Check sheet for the modelled part. Datum: model origin and axes. Units: mm. Face numbers are marked on the shaded views. A direction names the side the tool comes from. Round coordinates to 2 decimals unless told otherwise and drop trailing zeros. Loops run counter-clockwise (first coordinate to the right, second up) from the corner with the lowest first, then second, coordinate; pieces in that order, holes last. Notation, with made-up numbers: (2, -8) - (17, -8) arc R20 ccw to (17, 31) - close; hole circle Ø9 at (20.5, 36.5). An arc over 180 degrees is marked (long way). Return JSON: item names as keys, results as strings.
from build123d import *

# Parameters (mm, degrees)
REVOLVE1_ANGLE           = 180
BOSS_EXTRUDE1_REACH      = 58.967
BOSS_EXTRUDE1_END_RADIUS = 40
SKETCH3_R                = 5.5
CUT_EXTRUDE1_DEPTH       = 61.16851336
SKETCH4_R                = 3
CUT_EXTRUDE2_DEPTH       = 61.16851336
CUT_EXTRUDE3_DEPTH       = 61.093676973
CUT_EXTRUDE3_DEPTH_BACK  = 61.093676973
SKETCH5_W                = 18.19644254
SKETCH5_H                = 2.5
SKETCH5_W_2              = 19.029010645
CHAMFER1_SIZE            = 2
FILLET1_R                = 1


with BuildPart() as part:
    # Sketch1 → Revolve1 (revolve)
    with BuildSketch(Plane(origin=(0, 0, 0), x_dir=(1, 0, 0), z_dir=(0, 1, 0))):
        with BuildLine():
            Line((-20, 20.5), (-20, -20.5))
            Line((-20, -20.5), (-25, -20.5))
            Line((-25, -20.5), (-25, -17.5))
            Line((-25, -17.5), (-35.968736425, -17.5))
            ThreePointArc((-35.968736425, -17.5), (-40, 0), (-35.968736425, 17.5))
            Line((-35.968736425, 17.5), (-25, 17.5))
            Line((-25, 17.5), (-25, 20.5))
            Line((-25, 20.5), (-20, 20.5))
        make_face()
    revolve(axis=Axis((0, 0, 0), (0, 0, -1)), revolution_arc=REVOLVE1_ANGLE)

    # Boss-Extrude1: up to this sphere (the profile starts outside it)
    boss_extrude1_end = Location((0, 0, 0)) * Sphere(BOSS_EXTRUDE1_END_RADIUS, mode=Mode.PRIVATE)
    # Sketch2 → Boss-Extrude1 (add, up to the surface)
    with BuildSketch(Plane(origin=(0, 35, 0), x_dir=(-1, 0, 0), z_dir=(0, -1, 0)), mode=Mode.PRIVATE) as boss_extrude1_sk1:
        with BuildLine():
            Line((30, 9), (17.860571099, 9))
            ThreePointArc((17.860571099, 9), (20, 0), (17.860571099, -9))
            Line((17.860571099, -9), (30, -9))
            ThreePointArc((30, -9), (39, 0), (30, 9))
        make_face()
    boss_extrude1_tool1 = extrude(boss_extrude1_sk1.sketch, amount=BOSS_EXTRUDE1_REACH, mode=Mode.PRIVATE) - boss_extrude1_end
    boss_extrude1 = boss_extrude1_tool1.solids().sort_by_distance((-28.288022, 35, 0))[0]
    add(boss_extrude1)

    # Sketch3 → Cut-Extrude1 (cut, through all)
    with BuildSketch(Plane.XZ):
        with Locations(Location((-30, 0, 0), (0, 0, 270))):
            Circle(SKETCH3_R)
    cut_extrude1 = extrude(amount=-CUT_EXTRUDE1_DEPTH, mode=Mode.SUBTRACT)

    # Mirror1: Boss-Extrude1, Cut-Extrude1 across plane
    add(boss_extrude1.mirror(Plane(origin=(0, 0, 0), x_dir=(0, 0, 1), z_dir=(1, 0, 0))))
    add(cut_extrude1.mirror(Plane(origin=(0, 0, 0), x_dir=(0, 0, 1), z_dir=(1, 0, 0))), mode=Mode.SUBTRACT)

    # Sketch4 → Cut-Extrude2 (cut, through all)
    with BuildSketch(Plane.XZ):
        with Locations(Location((0, 0, 0), (0, 0, 270))):
            Circle(SKETCH4_R)
    extrude(amount=-CUT_EXTRUDE2_DEPTH, mode=Mode.SUBTRACT)

    # Sketch5 → Cut-Extrude3 (cut, two sides: drawn at the far end of the back side and taken through both)
    with BuildSketch(Plane.XY.offset(-CUT_EXTRUDE3_DEPTH_BACK)):
        with Locations((-39.09822127, 1.25)):
            Rectangle(SKETCH5_W, SKETCH5_H)
        with Locations((39.514505322, 1.25)):
            Rectangle(SKETCH5_W_2, SKETCH5_H)
    extrude(amount=CUT_EXTRUDE3_DEPTH + CUT_EXTRUDE3_DEPTH_BACK, mode=Mode.SUBTRACT)

    # Chamfer1
    chamfer1_edges = [part.edges().sort_by_distance(p)[0] for p in [
        (0, 20, -20.5),
        (0, 20, 20.5),
    ]]
    chamfer(chamfer1_edges, length=CHAMFER1_SIZE)

    # Fillet1
    fillet1_edges = [part.edges().sort_by_distance(p)[0] for p in [
        (0, 25, 20.5),
        (0, 25, 17.5),
        (0, 25, -17.5),
        (0, 25, -20.5),
    ]]
    fillet(fillet1_edges, radius=FILLET1_R)


solid = part.part
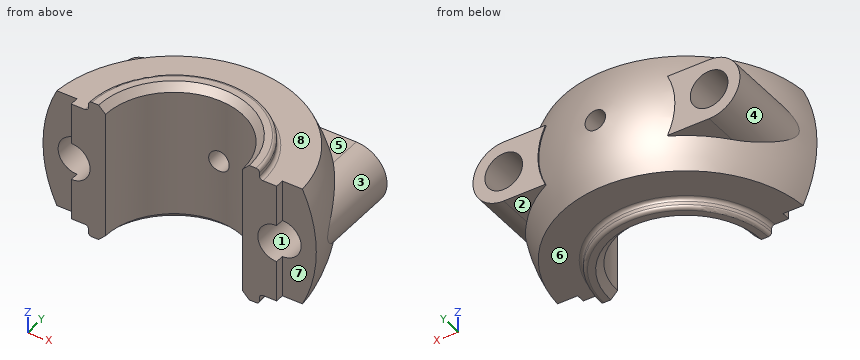
Q1. Sectioned sample at C-C (y = 14.5). State how many separate pieces and enclosed holes the cut face has, plus the area to 3 significant figures.
Answer key:
{"separate pieces": "2", "enclosed holes": "2", "area": "1,450 mm²"}
Q2. Sectioned sample at A-A (x = 0). Enter the section's corners in (y, z).
Answer key:
{"outline": "(20, -18.5) - (22, -20.5) - (24, -20.5) arc R1 ccw to (25, -19.5) - (25, -18.5) arc R1 cw to (26, -17.5) - (35.97, -17.5) arc R40 ccw to (39.89, -3) - (20, -3) - close; (20, 3) - (39.89, 3) arc R40 ccw to (35.97, 17.5) - (26, 17.5) arc R1 cw to (25, 18.5) - (25, 19.5) arc R1 ccw to (24, 20.5) - (22, 20.5) - (20, 18.5) - close"}
Q3. Sectioned sample at D-D (x = 31). Enter the section's corners in (y, z).
Answer key:
{"outline": "(2.5, -17.5) - (18.24, -17.5) arc R25.28 ccw to (23.64, -8.94) - (35, -8.94) - (35, -5.41) - (2.5, -5.41) - close; (2.5, 5.41) - (35, 5.41) - (35, 8.94) - (23.64, 8.94) arc R25.28 ccw to (18.24, 17.5) - (2.5, 17.5) - close"}
Q4. Tool access check on the marked faces 4, 5, 6, 7 and 8. Record the directions out of +Z, -Z, +X, -X, +Y, -Y that give a thin tool (end or side, any length) a straight path to the whole face; none if there is none.
Answer key:
{"face 4": "-X, +Y", "face 5": "+Z, +X, +Y", "face 6": "-Z, +Y", "face 7": "+Z, -Z, +X, -Y", "face 8": "+Z, +Y"}
Q5. Draft check along X on the marked faces 1, 2 and 3. Enter one of: released by +X, released by -X, zero draft, split by the parting line, or undercut.
Answer key:
{"face 1": "undercut", "face 2": "zero draft", "face 3": "released by +X"}
Q6. Scan lines: probe 1 along X at (y, z) = (28, 0); probe 2 along Z at (x, y) = (-30, 11); probe 3 along X at (y, z) = (28, 4). Record each from-to range of solid material in increasing order. Write a range as [from, to].
Answer key:
{"probe 1": "x = [-39, -35.5], [-24.5, -3], [3, 24.5], [35.5, 39]", "probe 2": "z = [-17.5, -5.5], [5.5, 17.5]", "probe 3": "x = [-38.06, -33.77], [-26.23, 26.23], [33.77, 38.06]"}
Q7. Depth check by flat-ended pin: P1, Ø5, axis at x = 14, z = 2.5, coming from the -Y side; P2, Ø8, axis at x = -36, z = 7, coming from the -Y side; P3, Ø8, axis at x = -23, y = 28.5, coming from the -Z side; P4, Ø6.5, axis at x = 30, z = 0, coming from the -Y side. Enter the tip coordinate at first touch or a pass-through.
Answer key:
{"P1": "stops at y = 11.3", "P2": "stops at y = 2.5", "P3": "stops at z = -17.5", "P4": "passes through"}
Q8. Sectioned sample at B-B (z = -11). Enter the section's corners in (x, y), plus the area to 3 significant figures.
Answer key:
{"outline": "(-38.38, 2.5) - (-30, 2.5) - (-30, 0) - (-20, 0) arc R20 cw to (20, 0) - (30, 0) - (30, 2.5) - (38.38, 2.5) arc R38.46 ccw to start", "area": "1,650 mm²"}
